Here's the drawing with two shaded views (mm, measured from the low corner). I have some questions. Round coordinates to 2 decimals unless told otherwise and drop trailing zeros. Order: outer loops, then holes, each group sorted by start corner. A loop starts at its lowest first (then second) coordinate and runs counter-clockwise, first axis right, second up.
Q1. We'd pull the mould along X, two halves only. Please class the marked faces 1, 2 and 3: pulls with the +X half, pulls with the -X half, needs draft (parallel to the pull), parting line crosses it, or undercut.
Q2. If I drill on line 1 (Z direction, x = 5.65, y = 0.8); line 2 (X direction, y = 2, z = 6); line 3 (Z direction, x = 1.5, y = 3.5), over which ranges is the centre line in solid material (lowest first)?
Q3. Will this pin go through, and if not, where does the flat tip stop? P1, Ø0.9, axis at x = 5.5, z = 5.5, coming from the -Y side.
Q4. If we section it at A-A (x = 5.65): Please give me the cut outline in (y, z).
Q5. If we section it at B-B (y = 8.5): Please give me the cut outline in (x, z), plus the area to 3 significant figures.
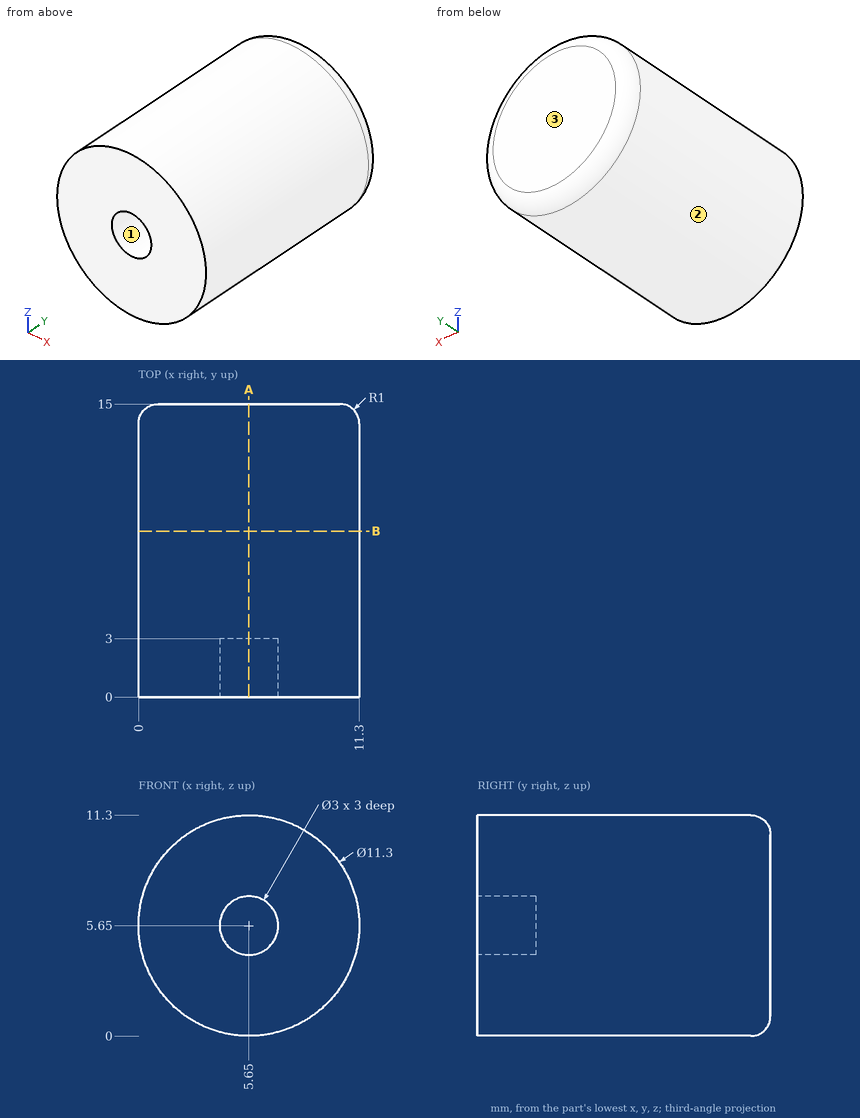
Solution:
1. face 1: undercut
1. face 2: parting line crosses it
1. face 3: needs draft
2. line 1: z = 0 to 4.15, 7.15 to 11.3
2. line 2: x = 0.01 to 4.19, 7.11 to 11.29
2. line 3: z = 1.82 to 9.48
3. P1: stops at y = 3
4. outline: (0, 0) - (14, 0) arc R1 ccw to (15, 1) - (15, 10.3) arc R1 ccw to (14, 11.3) - (0, 11.3) - (0, 7.15) - (3, 7.15) - (3, 4.15) - (0, 4.15) - close
5. outline: circle Ø11.3 at (5.65, 5.65)
5. area: 100 mm2
